from build123d import *

# Parameters (mm, degrees)
SKETCH1_W           = 440
SKETCH1_H           = 244
SKETCH1_W_2         = 60
SKETCH1_H_2         = 204
BOSS_EXTRUDE1_DEPTH = 5
BOSS_EXTRUDE2_DEPTH = 60
SKETCH3_W           = 65
SKETCH3_H           = 244
BOSS_EXTRUDE3_DEPTH = 10
SKETCH9_W           = 430
SKETCH9_H           = 5
BOSS_EXTRUDE6_DEPTH = 33
BOSS_EXTRUDE7_DEPTH = 38
SKETCH11_W          = 38
SKETCH11_H          = 33
CUT_EXTRUDE3_DEPTH  = 38
SKETCH12_W          = 13
SKETCH12_H          = 50
CUT_EXTRUDE4_DEPTH  = 10
CUT_EXTRUDE4_TAPER  = 30
CUT_EXTRUDE6_DEPTH  = 30
SKETCH16_W          = 5
SKETCH16_H          = 5
CUT_EXTRUDE7_DEPTH  = 435
SKETCH17_W          = 5
SKETCH17_H          = 234
BOSS_EXTRUDE8_DEPTH = 60
SKETCH18_W          = 210
SKETCH18_H          = 5
BOSS_EXTRUDE9_DEPTH = 60
SKETCH19_R          = 2.5
CUT_EXTRUDE8_DEPTH  = 50
SKETCH22_W          = 33
SKETCH22_H          = 5
CUT_EXTRUDE10_DEPTH = 150


with BuildPart() as part:
    # Sketch1 → Boss-Extrude1 (new body)
    with BuildSketch(Plane.XY):
        Rectangle(SKETCH1_W, SKETCH1_H)
        with Locations((-100, 0)):
            Rectangle(SKETCH1_W_2, SKETCH1_H_2, mode=Mode.SUBTRACT)
    extrude(amount=BOSS_EXTRUDE1_DEPTH)

    # Sketch2 → Boss-Extrude2 (add)
    with BuildSketch(Plane.XY.offset(5)):
        Polygon((-215, -117), (215, -117), (220, -122), (-220, -122), (-220, 122), (220, 122), (215, 117), (-215, 117), align=None)
    extrude(amount=BOSS_EXTRUDE2_DEPTH)

    # Sketch3 → Boss-Extrude3 (add)
    with BuildSketch(Plane.ZY.offset(220)):
        with Locations((32.5, 0)):
            Rectangle(SKETCH3_W, SKETCH3_H)
    extrude(amount=BOSS_EXTRUDE3_DEPTH)

    # Sketch9 → Boss-Extrude6 (add)
    with BuildSketch(Plane(origin=(0, -117, 0), x_dir=(1, 0, 0), z_dir=(0, 1, 0))):
        with Locations((0, -62.5)):
            Rectangle(SKETCH9_W, SKETCH9_H)
    boss_extrude6 = extrude(amount=BOSS_EXTRUDE6_DEPTH)

    # Sketch10 → Boss-Extrude7 (add)
    with BuildSketch(Plane.XY.offset(65)):
        Polygon((215, -84), (-215.042545238, -84), (-215.042545238, 122), (-230, 122), (-230, -89), (-215.042545238, -89), (215, -89), align=None)
    boss_extrude7 = extrude(amount=BOSS_EXTRUDE7_DEPTH)

    # Mirror4: Boss-Extrude6, Boss-Extrude7 across plane
    add(boss_extrude6.mirror(Plane.ZX))
    add(boss_extrude7.mirror(Plane.ZX))

    # Sketch11 → Cut-Extrude3 (cut)
    with BuildSketch(Plane(origin=(-215.042545238, 0, 0), x_dir=(0, 0, -1), z_dir=(1, 0, 0))):
        with Locations((-84, 105.5)):
            Rectangle(SKETCH11_W, SKETCH11_H)
        with Locations((-84, -105.5)):
            Rectangle(SKETCH11_W, SKETCH11_H)
    extrude(amount=-CUT_EXTRUDE3_DEPTH, mode=Mode.SUBTRACT)

    # Sketch12 → Cut-Extrude4 (cut)
    with BuildSketch(Plane.ZY.offset(230)):
        with Locations((38, 0)):
            Rectangle(SKETCH12_W, SKETCH12_H)
        with Locations((65, 0)):
            Rectangle(SKETCH12_W, SKETCH12_H)
    extrude(amount=-CUT_EXTRUDE4_DEPTH, taper=CUT_EXTRUDE4_TAPER, mode=Mode.SUBTRACT)

    # Sketch14 → Cut-Extrude6 (cut, symmetric)
    with BuildSketch(Plane(origin=(0, 0, 0), x_dir=(1, 0, 0), z_dir=(0, 1, 0))):
        Polygon((-230, -71.5), (-219.022191852, -54.5), (-230, -58.5), align=None)
        Polygon((-230, -31.5), (-219.022191852, -48.5), (-230, -44.5), align=None)
    extrude(amount=CUT_EXTRUDE6_DEPTH, both=True, mode=Mode.SUBTRACT)

    # Sketch16 → Cut-Extrude7 (cut)
    with BuildSketch(Plane(origin=(215, 0, 0), x_dir=(0, 0, -1), z_dir=(1, 0, 0))):
        with Locations((-100.5, -86.5)):
            Rectangle(SKETCH16_W, SKETCH16_H)
        with Locations((-100.5, 86.5)):
            Rectangle(SKETCH16_W, SKETCH16_H)
    extrude(amount=-CUT_EXTRUDE7_DEPTH, mode=Mode.SUBTRACT)

    # Sketch17 → Boss-Extrude8 (add)
    with BuildSketch(Plane.XY.offset(5)):
        with Locations((-67.5, 0)):
            Rectangle(SKETCH17_W, SKETCH17_H)
    extrude(amount=BOSS_EXTRUDE8_DEPTH)

    # Sketch18 → Boss-Extrude9 (add)
    with BuildSketch(Plane.XY.offset(5)):
        with Locations((35, 0)):
            Rectangle(SKETCH18_W, SKETCH18_H)
    extrude(amount=BOSS_EXTRUDE9_DEPTH)

    # Sketch19 → Cut-Extrude8 (cut)
    with BuildSketch(Plane.XY.offset(5)):
        with Locations((150, 0)):
            Circle(SKETCH19_R)
    extrude(amount=-CUT_EXTRUDE8_DEPTH, mode=Mode.SUBTRACT)

    # Sketch22 → Cut-Extrude10 (cut)
    with BuildSketch(Plane(origin=(215, 0, 0), x_dir=(0, 0, -1), z_dir=(1, 0, 0))):
        with Locations((-81.5, -86.5)):
            Rectangle(SKETCH22_W, SKETCH22_H)
        with Locations((-81.5, 86.5)):
            Rectangle(SKETCH22_W, SKETCH22_H)
    extrude(amount=-CUT_EXTRUDE10_DEPTH, mode=Mode.SUBTRACT)


solid = part.part
The listing builds one solid part. Answer for the finished solid, in the listing's coordinates (mm). A direction names the side the tool comes from. Give positions to 0.01 mm unless a question says otherwise; leave off trailing zeros. Write each loop counter-clockwise with the first axis right and the second up, starting at its lowest first coordinate (ties: lowest second). Pieces come first, ordered by that corner, then holes.
1) Section D-D (x = 107.5) is taken. Write down the section's boundary in (y, z).
2) Given P1, Ø6, axis at y = -22, z = 52, coming from the +X side; P2, Ø3, axis at y = 27, z = 88.5, coming from the +X side; P3, Ø5.5, axis at y = -94.5, z = 63.5, coming from the +X side, each flat-ended and moving along its own axis, determine where each tip first touches the part or whether it passes through.
3) Find the intervals of material crossed by L1, parallel to Y at x = 27.5, z = 48; L2, parallel to Y at x = 150, z = 2.9; L3, parallel to X at y = -22, z = 22, in increasing order.
4) Section C-C (z = 92.5) is taken. Write down the section's boundary in (x, y), and give its area (3 significant figures).
5) Section A-A (x = -85) is taken. Write down the section's boundary in (y, z).
6) For a pull along X with two mould halves and no side action, classify faces 5 (the face through (-215.043, -1, 84)), 6 (the face through (77, 117, 32)), 7 (the face through (-144, 101, 60)) as pulls with the +X half, pulls with the -X half, needs draft (parallel to the pull), parting line crosses it, or undercut.
7) Section B-B (y = -67.5) is taken. Write down the section's boundary in (x, z), and give its area (3 significant figures).
8) A tool of negligible diameter and unlimited length cuts with its end or side. For faces 1 (the face through (-12, 0, 65)), 2 (the face through (-85, 89, 80)), 3 (the face through (-80, -89, 84)), 4 (the face through (-215, 2, 35)), from which of +Z, -Z, +X, -X, +Y, -Y can it reach the whole face along a straight path? Write none if from no direction.
Response:
1. outline: (-122, 0) - (122, 0) - (122, 65) - (84, 65) - (84, 60) - (117, 60) - (117, 5) - (2.5, 5) - (2.5, 65) - (-2.5, 65) - (-2.5, 5) - (-117, 5) - (-117, 60) - (-84, 60) - (-84, 65) - (-122, 65) - close
2. P1: stops at x = -65
2. P2: stops at x = -215.04
2. P3: stops at x = 215
3. L1: y = -122 to -117, -2.5 to 2.5, 117 to 122
3. L2: y = -122 to -2.5, 2.5 to 122
3. L3: x = -230 to -215, -70 to -65
4. outline: (-230, -89) - (65, -89) - (65, -84) - (-215.04, -84) - (-215.04, 84) - (65, 84) - (65, 89) - (-230, 89) - close
4. area: 5,460 mm2
5. outline: (-122, 0) - (-102, 0) - (-102, 5) - (-117, 5) - (-117, 60) - (-84, 60) - (-84, 98) - (-89, 98) - (-89, 65) - (-122, 65) - close; (84, 60) - (117, 60) - (117, 5) - (102, 5) - (102, 0) - (122, 0) - (122, 65) - (89, 65) - (89, 98) - (84, 98) - close
6. face 5: pulls with the +X half
6. face 6: needs draft
6. face 7: undercut
7. outline: (-230, 0) - (-130, 0) - (-130, 5) - (-215, 5) - (-215, 65) - (-215.04, 65) - (-215.04, 103) - (-230, 103) - close; (-70, 0) - (220, 0) - (220, 5) - (-65, 5) - (-65, 65) - (-70, 65) - close
7. area: 3,720 mm2
8. face 1: +Z, +X
8. face 2: +Z, +X, -X, +Y
8. face 3: +Z, +X, -X, -Y
8. face 4: none
